Could you check a few things on this model? Use its own coordinates, in mm. Face numbers are marked on the shaded views. A direction names the side the tool comes from. Give positions to 0.01 mm unless a question says otherwise; leave off trailing zeros. Loops run counter-clockwise (first coordinate to the right, second up) from the corner with the lowest first, then second, coordinate; pieces in that order, holes last. Notation, with made-up numbers: M 20,60 L 60,60 A33 cw 60,96 Z; hole C -14.75,-22.75 d6. An arc over 180 degrees is marked long. Use a Markdown table: item, result. Add a question column.
1) Suppose I cut it at A-A on z = -0.25. List the corners of the cut face in (x, y) for me, and give its area (3 significant figures).
2) If I drill on line 1 along X through (y, z) = (5.25, -2.75); line 2 along Z through (x, y) = (8.25, 2.5); line 3 along Z through (x, y) = (8.25, 8.25), over which ranges is the centre line in solid material (lowest first)? Write a range as [from, to].
3) Suppose I cut it at B-B on z = 5. List the corners of the cut face in (x, y) for me, and give its area (3 significant figures).
4) Which directions (+Z, -Z, +X, -X, +Y, -Y) give clear straight access to the entire face, cutting with the end or side of a thin tool? Please do the marked faces 1, 2, 3 and 4.
5) Suppose I cut it at D-D on y = 8. List the corners of the cut face in (x, z) for me.
6) Will these pins go through, and if not, where does the flat tip stop? pin 1 Ø2 at (x, z) = (3, -1.5) entering from -Y; pin 2 Ø1.8 at (x, z) = (8, 5.5) entering from -Y; pin 3 Ø0.9 at (y, z) = (5, -2.5) entering from -X.
7) We'd pull the mould along Y, two halves only. Please class the marked faces 5, 6, 7 and 8: +Y half, -Y half, draft (parallel to the pull), parting line (faces both ways), or undercut.
8) Suppose I cut it at C-C on x = 5. List the corners of the cut face in (y, z) for me.
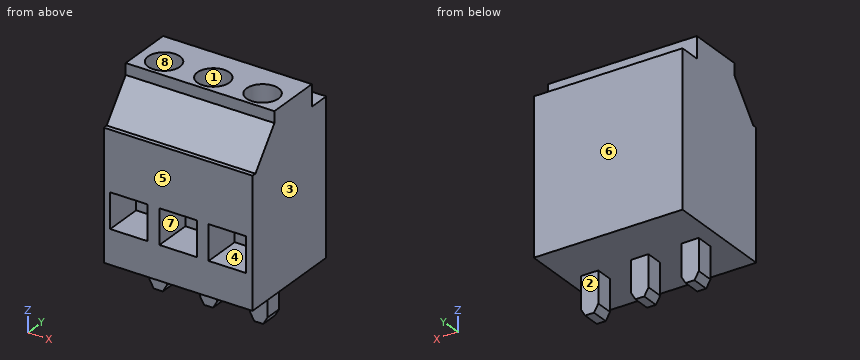
```python
from build123d import *
from OCP.BRepFilletAPI import BRepFilletAPI_MakeChamfer

# Parameters (mm, degrees)
SKETCH1_W           = 15.34
SKETCH1_H           = 11.35
BOSS_EXTRUDE1_DEPTH = 18
SKETCH1_3_W         = 1.8
SKETCH1_3_H         = 1.8
BOSS_EXTRUDE2_DEPTH = 4
CHAMFER1_SIZE       = 0.762
CHAMFER1_SIZE2      = 0.439940905
SKETCH3_W           = 2.211259549
SKETCH3_H           = 2.211259549
CUT_EXTRUDE1_DEPTH  = 27.232386472
SKETCH4_R           = 1.650097839
CUT_EXTRUDE2_DEPTH  = 4
SKETCH2_W           = 3.858538726
SKETCH2_H           = 3.6
CUT_EXTRUDE3_DEPTH  = 4


with BuildPart() as part:
    # Sketch1 → Boss-Extrude1 (new body)
    with BuildSketch(Plane.XY):
        with Locations((7.67, 5.675)):
            Rectangle(SKETCH1_W, SKETCH1_H)
    extrude(amount=BOSS_EXTRUDE1_DEPTH)

    # Sketch1<3> → Boss-Extrude2 (add)
    with BuildSketch(Plane.XY):
        with Locations((2.54, 5.5)):
            Rectangle(SKETCH1_3_W, SKETCH1_3_H)
        with Locations((7.72, 5.5)):
            Rectangle(SKETCH1_3_W, SKETCH1_3_H)
        with Locations((12.9, 5.5)):
            Rectangle(SKETCH1_3_W, SKETCH1_3_H)
    extrude(amount=-BOSS_EXTRUDE2_DEPTH)

    # Chamfer1: one chamfer whose edges measure the first distance from different faces: ONE call of the kernel's chamfer builder (chamfer() names one face for all edges)
    chamfer1_edges_1 = [part.edges().sort_by_distance(p)[0] for p in [
        (1.64, 5.5, -4),
    ]]
    chamfer1_side_1 = [part.faces().sort_by_distance(p)[0] for p in [
        (1.64, 5.5, -2),
    ]]
    chamfer1_edges_2 = [part.edges().sort_by_distance(p)[0] for p in [
        (3.44, 5.5, -4),
    ]]
    chamfer1_side_2 = [part.faces().sort_by_distance(p)[0] for p in [
        (3.44, 5.5, -2),
    ]]
    chamfer1_edges_3 = [part.edges().sort_by_distance(p)[0] for p in [
        (6.82, 5.5, -4),
    ]]
    chamfer1_side_3 = [part.faces().sort_by_distance(p)[0] for p in [
        (6.82, 5.5, -2),
    ]]
    chamfer1_edges_4 = [part.edges().sort_by_distance(p)[0] for p in [
        (8.62, 5.5, -4),
    ]]
    chamfer1_side_4 = [part.faces().sort_by_distance(p)[0] for p in [
        (8.62, 5.5, -2),
    ]]
    chamfer1_edges_5 = [part.edges().sort_by_distance(p)[0] for p in [
        (12, 5.5, -4),
    ]]
    chamfer1_side_5 = [part.faces().sort_by_distance(p)[0] for p in [
        (12, 5.5, -2),
    ]]
    chamfer1_edges_6 = [part.edges().sort_by_distance(p)[0] for p in [
        (13.8, 5.5, -4),
    ]]
    chamfer1_side_6 = [part.faces().sort_by_distance(p)[0] for p in [
        (13.8, 5.5, -2),
    ]]
    chamfer1 = BRepFilletAPI_MakeChamfer(part.part.solid().wrapped)
    for e in chamfer1_edges_1:
        chamfer1.Add(CHAMFER1_SIZE, CHAMFER1_SIZE2, e.wrapped, chamfer1_side_1[0].wrapped)  # the first distance lies on this face
    for e in chamfer1_edges_2:
        chamfer1.Add(CHAMFER1_SIZE, CHAMFER1_SIZE2, e.wrapped, chamfer1_side_2[0].wrapped)  # the first distance lies on this face
    for e in chamfer1_edges_3:
        chamfer1.Add(CHAMFER1_SIZE, CHAMFER1_SIZE2, e.wrapped, chamfer1_side_3[0].wrapped)  # the first distance lies on this face
    for e in chamfer1_edges_4:
        chamfer1.Add(CHAMFER1_SIZE, CHAMFER1_SIZE2, e.wrapped, chamfer1_side_4[0].wrapped)  # the first distance lies on this face
    for e in chamfer1_edges_5:
        chamfer1.Add(CHAMFER1_SIZE, CHAMFER1_SIZE2, e.wrapped, chamfer1_side_5[0].wrapped)  # the first distance lies on this face
    for e in chamfer1_edges_6:
        chamfer1.Add(CHAMFER1_SIZE, CHAMFER1_SIZE2, e.wrapped, chamfer1_side_6[0].wrapped)  # the first distance lies on this face
    add(Compound.cast(chamfer1.Shape()), mode=Mode.REPLACE)

    # Sketch3 → Cut-Extrude1 (cut, through all)
    with BuildSketch(Plane.ZY):
        with Locations((16.894370226, 10.244370226)):
            Rectangle(SKETCH3_W, SKETCH3_H)
        Polygon((18, 0), (18, 3.37428008), (16.831701498, 3.37428008), (13.224191742, 0.450816104), (13.224191742, 0), align=None)
    extrude(amount=-CUT_EXTRUDE1_DEPTH, mode=Mode.SUBTRACT)

    # Sketch4 → Cut-Extrude2 (cut)
    with BuildSketch(Plane.XY.offset(18)):
        with Locations((2.59, 5.419196483)):
            Circle(SKETCH4_R)
        with Locations((7.67, 5.419196483)):
            Circle(SKETCH4_R)
        with Locations((12.75, 5.419196483)):
            Circle(SKETCH4_R)
    extrude(amount=-CUT_EXTRUDE2_DEPTH, mode=Mode.SUBTRACT)

    # Sketch2 → Cut-Extrude3 (cut)
    with BuildSketch(Plane.XZ):
        with Locations((2.59, 5.3)):
            Rectangle(SKETCH2_W, SKETCH2_H)
        with Locations((7.67, 5.3)):
            Rectangle(SKETCH2_W, SKETCH2_H)
        with Locations((12.75, 5.3)):
            Rectangle(SKETCH2_W, SKETCH2_H)
    extrude(amount=-CUT_EXTRUDE3_DEPTH, mode=Mode.SUBTRACT)


solid = part.part
```
Answer block:
| question | item | result |
|---|---|---|
| 1 | outline | M 1.64,4.6 L 3.44,4.6 L 3.44,6.4 L 1.64,6.4 Z; M 6.82,4.6 L 8.62,4.6 L 8.62,6.4 L 6.82,6.4 Z; M 12,4.6 L 13.8,4.6 L 13.8,6.4 L 12,6.4 Z |
| 1 | area | 9.72 mm^2 |
| 2 | line 1 | x = [1.64, 3.44], [6.82, 8.62], [12, 13.8] |
| 2 | line 2 | z = [0, 3.5], [7.1, 15.75] |
| 2 | line 3 | z = [0, 18] |
| 3 | outline | M 0,0 L 0.66,0 L 0.66,4 L 4.52,4 L 4.52,0 L 5.74,0 L 5.74,4 L 9.6,4 L 9.6,0 L 10.82,0 L 10.82,4 L 14.68,4 L 14.68,0 L 15.34,0 L 15.34,11.35 L 0,11.35 Z |
| 3 | area | 128 mm^2 |
| 4 | face 1 | +Z |
| 4 | face 2 | -Z, +X, -X, +Y |
| 4 | face 3 | +Z, -Z, +X, +Y, -Y |
| 4 | face 4 | -Y |
| 5 | outline | M 0,0 L 15.34,0 L 15.34,18 L 0,18 Z |
| 6 | pin 1 | stops at y = 4.6 |
| 6 | pin 2 | stops at y = 4 |
| 6 | pin 3 | stops at x = 1.64 |
| 7 | face 5 | -Y half |
| 7 | face 6 | +Y half |
| 7 | face 7 | draft |
| 7 | face 8 | undercut |
| 8 | outline | M 0,0 L 11.35,0 L 11.35,15.79 L 9.14,15.79 L 9.14,18 L 3.37,18 L 3.37,16.83 L 0.45,13.22 L 0,13.22 Z |
